Autodesk Inventor part; units mm, degrees
ref_plane "YZ Plane" through (0, 0, 0) normal (1, 0, 0) x (0, 1, 0)
ref_plane "XZ Plane" through (0, 0, 0) normal (0, 1, 0) x (-1, 0, 0)
ref_plane "XY Plane" through (0, 0, 0) normal (0, 0, 1) x (1, 0, 0)
sketch "Skizze1" plane through (0, 0, 0) normal (0, 0, 1) x (1, 0, 0)
  circle A0 centre (0, 0) radius 24.4
  dimension "d0" = 48.8
extrude "Extrusion1" add sketch "Skizze1" along normal blind 9
sketch "Skizze2" plane through (0, 0, 9) normal (0, 0, 1) x (1, 0, 0)
  circle A0 centre (0, 0) radius 24.4
  circle A1 centre (0, 0) radius 11.5
  dimension "d5" = 23
extrude "Extrusion2" cut sketch "Skizze2" against normal blind 1.5 contours A1
sketch "Skizze10" plane through (0, 0, 9) normal (0, 0, 1) x (1, 0, 0)
  circle A0 centre (0, 0) radius 24.4
  circle A1 centre (0, 0) radius 23.75
  dimension "d62" = 47.5
extrude "Extrusion3" cut sketch "Skizze10" against normal blind 7
sketch "Skizze12" plane through (0, 0, 0) normal (0, 0, -1) x (-1, 0, 0)
  circle A0 centre (0, 0) radius 24.4
  circle A1 centre (0, 0) radius 23.5
  dimension "d82" = 47
extrude "Extrusion4" [suppressed]
sketch "Skizze5" plane through (0, 0, 9) normal (0, 0, 1) x (1, 0, 0)
  circle A0 centre (0, 0) radius 11.5
  circle A1 centre (0, 0) radius 24.4
  circle A2 centre (0, 0) radius 17.5
  point P0 (0, 17.5)
  point P1 (0, -17.5)
  dimension "d17" = 35
hole "Bohrung2" at (0, 17.5, 9) at (0, -17.5, 9) direction (0, 0, -1) diameter 3 end through all
sketch "Skizze6" plane through (0, 0, 9) normal (0, 0, 1) x (1, 0, 0)
  circle A0 centre (0, 17.5) radius 1.5
  circle A1 centre (0, -17.5) radius 1.5
  circle A2 centre (0, 0) radius 11.5
  circle A3 centre (0, 0) radius 24.4
  circle A4 centre (0, 17.5) radius 1.5
  circle A5 centre (0, -17.5) radius 1.5
  circle A6 centre (0, 0) radius 11.5
  circle A7 centre (0, 0) radius 17.5
  point P0 (5.9854, 16.4446)
  point P1 (-5.9854, -16.4446)
  dimension "d25" = 20
  dimension "d26" = 20
hole "Bohrung3" at (5.9854, 16.4446, 9) at (-5.9854, -16.4446, 9) direction (0, 0, -1) diameter 2.459 end through all
sketch "Skizze4" plane through (0, 0, 7.5) normal (0, 0, 1) x (1, 0, 0)
  circle A0 centre (0, 0) radius 11.5
  circle A1 centre (0, 0) radius 6.35
  circle A2 centre (5.9854, 16.4446) radius 1.2295
  circle A3 centre (-5.9854, -16.4446) radius 1.2295
  line L0 (5.9854, 16.4446) -> (-5.9854, -16.4446)
  line L1 (-8.743, 3.1822) -> (10.8065, -3.9332)
  point P0 (5.967, -2.1718)
  point P1 (-5.967, 2.1718)
  dimension "d9" = 12.7
hole "Bohrung1" at (5.967, -2.1718, 7.5) at (-5.967, 2.1718, 7.5) direction (0, 0, -1) diameter 1.567 end through all
chamfer "Fase3" distance 1 angle 45 1 edges at (-23.75, 0, 9)
chamfer "Fase6" [suppressed]
sketch "Skizze15" plane through (0, 0, 9) normal (0, 0, 1) x (1, 0, 0)
  circle A0 centre (0, 0) radius 10 construction
  line L0 (-6.4279, 7.6604) -> (7.0707, -8.4265) construction
  line L1 (0, -34.16) -> (0, 34.16) construction
  line L2 (0, 0) -> (11, 0) construction
  point P0 (6.4279, -7.6604)
  dimension "d110" = 20
  dimension "d111" = 40
  dimension "d115" = 11
hole "Bohrung9" at (6.4279, -7.6604, 9) at (-6.4279, 7.6604, 9) direction (0, 0, -1) diameter 3 end through all
sketch "Skizze17" plane through (0, 0, 0) normal (0, 0, -1) x (-1, 0, 0)
  circle A0 centre (0, 0) radius 18 construction
  circle A1 centre (0, 0) radius 23.75 construction
  line L0 (11.5702, 13.7888) -> (-11.5702, -13.7888) construction
  point P0 (7.3921, 8.8095)
  point P1 (-7.3921, -8.8095)
  dimension "d134" = 36
hole "Bohrung11" at (11.5702, -13.7888, 0) at (-11.5702, 13.7888, 0) direction (0, 0, 1) diameter 2.459 end through all
properties part number "Ledaufnahme"
CAD build for the part. Positions are in the model's coordinates, mm. A direction names the side the tool comes from. Coordinates: 2 decimals unless noted, no trailing zeros. Order: outer loops, then holes, each group sorted by start corner. A loop starts at its lowest first (then second) coordinate and runs counter-clockwise, first axis right, second up.
(1) Saw through at B-B, the plane z = 1. Count the separate pieces of the cut face and the enclosed holes in it, and give its area (3 significant figures).
Solution:
separate pieces: 1
enclosed holes: 10
area: 1,820 mm2
(2) Saw through at A-A, the plane x = 0. Write the cut outline in (y, z), and give its area (3 significant figures).
Solution:
outline: (-24.4, 0) - (-19, 0) - (-19, 9) - (-22.75, 9) - (-23.75, 8) - (-23.75, 2) - (-24.4, 2) - close; (-16, 0) - (16, 0) - (16, 9) - (11.5, 9) - (11.5, 7.5) - (-11.5, 7.5) - (-11.5, 9) - (-16, 9) - close; (19, 0) - (24.4, 0) - (24.4, 2) - (23.75, 2) - (23.75, 8) - (22.75, 9) - (19, 9) - close
area: 341 mm2
(3) Which spindle directions (+Z, -Z, +X, -X, +Y, -Y) get a long thin tool onto all of the face, cutting with end or side? Do faces 1 (the face through (-1.5, 11.4, 8.3)), 2 (the face through (6, -9.1, 3.7)). Say none if no direction does.
Solution:
face 1: +Z
face 2: +Z, -Z
(4) Saw through at C-C, the plane y = 0. Write the cut outline in (x, z), and give its area (3 significant figures).
Solution:
outline: (-24.4, 0) - (24.4, 0) - (24.4, 2) - (23.75, 2) - (23.75, 8) - (22.75, 9) - (11.5, 9) - (11.5, 7.5) - (-11.5, 7.5) - (-11.5, 9) - (-22.75, 9) - (-23.75, 8) - (-23.75, 2) - (-24.4, 2) - close
area: 395 mm2
(5) Pin check, flat tips, straight feed: pin 1 Ø3 at (x, z) = (12, 2.5) entering from +Y; pin 2 Ø1 at (x, z) = (18.5, 5) entering from -Y; pin 3 Ø1 at (y, z) = (-3, 1) entering from +X. Stop position of each tip, or through.
Solution:
pin 1: stops at y = 21.98
pin 2: stops at y = -15.49
pin 3: stops at x = 24.27
(6) Mould opens along X. For faces 3 (the face through (-11.94, 14.96, 4.56)), 4 (the face through (-24.376, -1.073, 0.986)), 5 (the face through (5.3, -23.4, 2)) say: released by +X, released by -X, zero draft, split by the parting line, or undercut.
Solution:
face 3: undercut
face 4: split by the parting line
face 5: zero draft
(7) Drill centre lines: L1, parallel to Y at x = 0, z = 6.75; L2, parallel to Y at x = 0, z = 7.9; L3, parallel to Y at x = 1, z = 7.25. Where is each one in solid material? Low to high.
Solution:
L1: y = -23.75 to -19, -16 to 16, 19 to 23.75
L2: y = -23.75 to -19, -16 to -11.5, 11.5 to 16, 19 to 23.75
L3: y = -23.73 to -18.62, -16.38 to 16.38, 18.62 to 23.73
